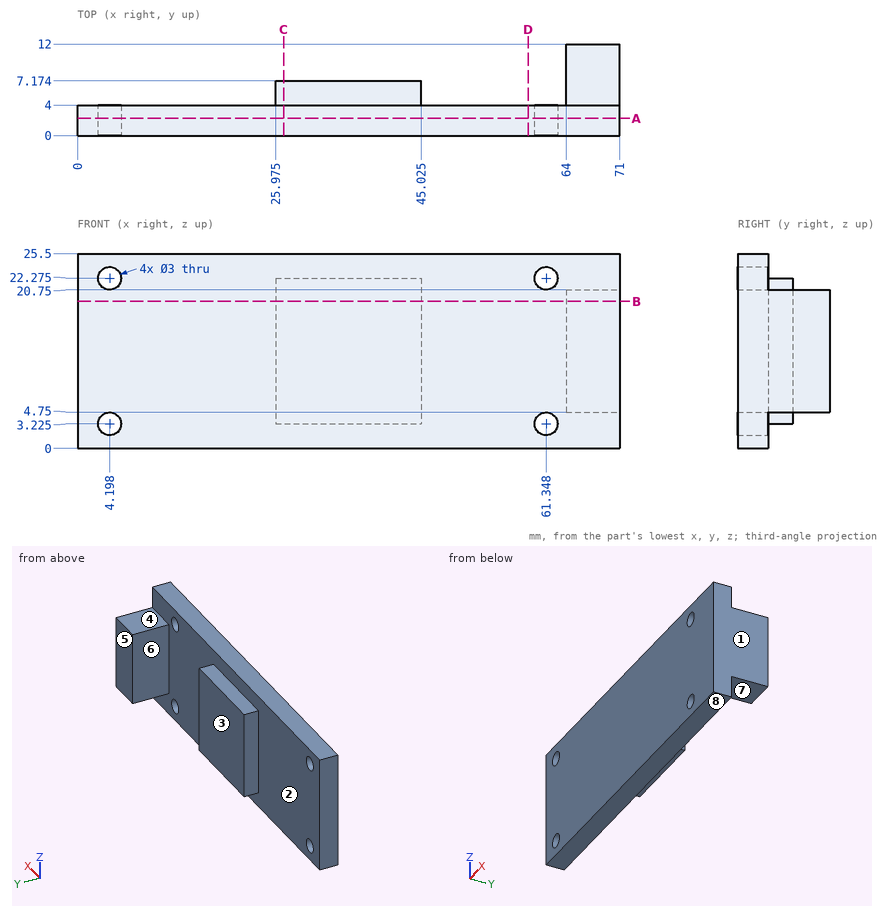
Here's the drawing with two shaded views (mm, measured from the low corner). I have some questions. A direction names the side the tool comes from. Round coordinates to 2 decimals unless told otherwise and drop trailing zeros. Loops run counter-clockwise (first coordinate to the right, second up) from the corner with the lowest first, then second, coordinate; pieces in that order, holes last. Notation, with made-up numbers: (36, 17) -> (55, 17) arc R33 ccw to (55, 53) -> close; hole circle Ø8 at (36.5, 58). An arc over 180 degrees is marked (long way). Answer as CSV lines item,"result". Start each with the question number.
1. Imagine slicing it at B-B on z = 19.25. Write out the boundary of the cut face in (x, y) (3 decimals).
2. I need wall thicknesses on probe 1 along X at (y, z) = (4.5, 5.75) (3 decimals); probe 2 along X at (y, z) = (1, 4); probe 3 along X at (y, z) = (2, 3.25). Which ranges of each line are inside material? Lowest first, please. Write a range as from..to.
3. For the marked faces 4, 5, 6, 7 and 8, which set-ups out of +Z, -Z, +X, -X, +Y, -Y let a thin tool reach every point of the face, with its end or its side?
4. I'm going to push flat-ended pins straight in: P1, Ø2, axis at x = 66, y = 7.5, coming from the +Z side; P2, Ø5.5, axis at x = 68.5, y = 9, coming from the -Z side; P3, Ø5.5, axis at x = 35.5, z = 16.5, coming from the +Y side. Where does each tip first touch, or does it pass through?
5. Imagine slicing it at D-D on x = 59. Write out the boundary of the cut face in (y, z).
6. If we mould it in two halves opening along X, with no side actions, what happens to the marked faces 1, 2 and 3? For each: pulls with the +X half, pulls with the -X half, needs draft (parallel to the pull), parting line crosses it, or undercut.
7. Imagine slicing it at C-C on x = 27. Write out the boundary of the cut face in (y, z) (3 decimals), plus the area to 3 significant figures.
8. Imagine slicing it at A-A on y = 2.25. Write out the boundary of the cut face in (x, z) (3 decimals).
Solution:
1,outline,"(0, 0) -> (71, 0) -> (71, 12) -> (64, 12) -> (64, 4) -> (45.025, 4) -> (45.025, 7.174) -> (25.975, 7.174) -> (25.975, 4) -> (0, 4) -> close"
2,probe 1,"25.975..45.025, 64..71"
2,probe 2,"0..2.91, 5.48..60.06, 62.63..71"
2,probe 3,"0..2.7, 5.7..59.85, 62.85..71"
3,face 4,"+Z, +X, +Y"
3,face 5,"+Z, -Z, +X, -X, +Y"
3,face 6,"+Z, -Z, +Y"
3,face 7,"-Z, +X, +Y"
3,face 8,"-Z, +X, -X, +Y, -Y"
4,P1,"z = 20.75"
4,P2,"z = 4.75"
4,P3,"y = 7.17"
5,outline,"(0, 0) -> (4, 0) -> (4, 25.5) -> (0, 25.5) -> close"
6,face 1,"pulls with the +X half"
6,face 2,"undercut"
6,face 3,"needs draft"
7,outline,"(0, 0) -> (4, 0) -> (4, 3.225) -> (7.174, 3.225) -> (7.174, 22.275) -> (4, 22.275) -> (4, 25.5) -> (0, 25.5) -> close"
7,area,"162 mm²"
8,outline,"(0, 0) -> (71, 0) -> (71, 25.5) -> (0, 25.5) -> close; hole circle Ø3 at (4.198, 3.225); hole circle Ø3 at (4.198, 22.275); hole circle Ø3 at (61.348, 3.225); hole circle Ø3 at (61.348, 22.275)"
